Can you work these out from the model? Positions are in its coordinate system, mm. Give positions to 0.01 mm unless a question says otherwise; leave off trailing zeros. Write each loop counter-clockwise with the first axis right and the second up, starting at its lowest first coordinate (ties: lowest second). Pieces come first, ordered by that corner, then holes. Notation, with made-up numbers: (6.25, -20) -> (32.25, -20) arc R28 ccw to (32.25, 12) -> close; hole circle Ø5 at (21, -39.75). An arc over 180 degrees is marked (long way). One line per item, written item: value.
Autodesk Inventor part; units mm, degrees
ref_plane "YZ Plane" through (0, 0, 0) normal (1, 0, 0) x (0, 1, 0)
ref_plane "XZ Plane" through (0, 0, 0) normal (0, 1, 0) x (-1, 0, 0)
ref_plane "XY Plane" through (0, 0, 0) normal (0, 0, 1) x (1, 0, 0)
sketch "Sketch1" plane through (0, 0, 0) normal (0, 0, 1) x (1, 0, 0)
  arc A0 (145.923, -27.051) -> (149.098, -23.876) centre (145.923, -23.876) ccw
  line L0 (149.098, -1.3151) -> (149.098, -23.876)
  line L1 (0, -23.876) -> (0, -1.3151)
  line L2 (148.1681, 0.9299) -> (76.7941, 72.3039)
  line L3 (0.9299, 0.9299) -> (72.3039, 72.3039)
  circle A1 centre (25.4, 0) radius 2.2098
  circle A2 centre (123.698, 0) radius 2.2098
  arc A3 (0, -23.876) -> (3.175, -27.051) centre (3.175, -23.876) ccw
  arc A4 (76.7941, 72.3039) -> (72.3039, 72.3039) centre (74.549, 70.0589) ccw
  arc A5 (0.9299, 0.9299) -> (0, -1.3151) centre (3.175, -1.3151) ccw
  arc A6 (149.098, -1.3151) -> (148.1681, 0.9299) centre (145.923, -1.3151) ccw
  line L4 (74.549, 73.2339) -> (74.549, -27.051)
  line L5 (145.923, -27.051) -> (3.175, -27.051)
  point P0 (0, 0)
  point P1 (76.7941, 72.3039)
  point P2 (0, -1.3151)
  point P3 (74.549, 23.0914)
  point P4 (3.175, -27.051)
extrude "Extrusion1" add sketch "Sketch1" along normal blind 1.5875
properties part number "alignernew"
1) If we section it at B-B (z = 1.3): Write out the boundary of the cut face in (x, y) (3 decimals).
Answer list:
outline: (0, -23.876) arc R3.175 ccw to (3.175, -27.051) -> (145.923, -27.051) arc R3.175 ccw to (149.098, -23.876) -> (149.098, -1.315) arc R3.175 ccw to (148.168, 0.93) -> (76.794, 72.304) arc R3.175 ccw to (72.304, 72.304) -> (0.93, 0.93) arc R3.175 ccw to (0, -1.315) -> close; hole circle Ø4.42 at (25.4, 0); hole circle Ø4.42 at (123.698, 0)
2) If we section it at D-D (y = 33): Write out the boundary of the cut face in (x, z).
Answer list:
outline: (33, 0) -> (116.1, 0) -> (116.1, 1.59) -> (33, 1.59) -> close
3) We'd pull the mould along X, two halves only. Please class faces 1 (the face through (27.44, 0.85, 0.78)), 2 (the face through (74, 13, 1.588)), 3 (the face through (148.19, -26.1, 0.78)): released by +X, released by -X, zero draft, split by the parting line, or undercut.
Answer list:
face 1: undercut
face 2: zero draft
face 3: released by +X
4) If we section it at A-A (x = 25.4): Write out the boundary of the cut face in (y, z).
Answer list:
outline: (-27.05, 0) -> (-2.21, 0) -> (-2.21, 1.59) -> (-27.05, 1.59) -> close; (2.21, 0) -> (25.4, 0) -> (25.4, 1.59) -> (2.21, 1.59) -> close
5) If we section it at C-C (x = 57): Write out the boundary of the cut face in (y, z), and give its area (3 significant figures).
Answer list:
outline: (-27.05, 0) -> (57, 0) -> (57, 1.59) -> (-27.05, 1.59) -> close
area: 133 mm^2
6) I need wall thicknesses on L1, parallel to X at y = -2, z = 1.25; L2, parallel to X at y = 65, z = 1.3; L3, parallel to Y at x = 25.4, z = 1.15. Which ranges of each line are inside material? Lowest first, please.
Answer list:
L1: x = 0 to 24.46, 26.34 to 122.76, 124.64 to 149.1
L2: x = 65 to 84.1
L3: y = -27.05 to -2.21, 2.21 to 25.4
